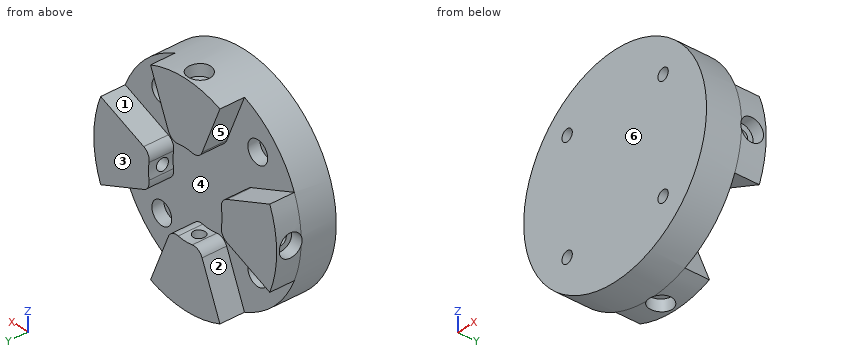
```python
from build123d import *

# Parameters (mm, degrees)
SKETCH1_R                                           = 30
BOSS_EXTRUDE1_DEPTH                                 = 10
CBORE_FOR_M3_HEX_SOCKET_HEAD_CAP_SCREW1_D           = 3.4
CBORE_FOR_M3_HEX_SOCKET_HEAD_CAP_SCREW1_CBORE_D     = 6.5
CBORE_FOR_M3_HEX_SOCKET_HEAD_CAP_SCREW1_CBORE_DEPTH = 3.4
BOSS_EXTRUDE2_DEPTH                                 = 7
CBORE_FOR_M3_HEX_SOCKET_HEAD_CAP_SCREW2_D           = 3.4
CBORE_FOR_M3_HEX_SOCKET_HEAD_CAP_SCREW2_DEPTH       = 18.91444561
CBORE_FOR_M3_HEX_SOCKET_HEAD_CAP_SCREW2_CBORE_D     = 6.5
CBORE_FOR_M3_HEX_SOCKET_HEAD_CAP_SCREW2_CBORE_DEPTH = 3.4
CIRPATTERN1_COUNT                                   = 4
FILLET1_R                                           = 3
CUT_EXTRUDE1_REACH                                  = 47.706
CIRPATTERN2_COUNT                                   = 4


with BuildPart() as part:
    # Sketch1 → Boss-Extrude1 (new body)
    with BuildSketch(Plane(origin=(0, 0, 0), x_dir=(1, 0, 0), z_dir=(0, 1, 0))):
        with Locations(Location((0, 0, 0), (0, 0, 270))):
            Circle(SKETCH1_R)
    extrude(amount=BOSS_EXTRUDE1_DEPTH)

    # CBORE for M3 Hex Socket Head Cap Screw1 (through all)
    with Locations(Plane(origin=(0, 10, 0), x_dir=(1, 0, 0), z_dir=(0, 1, 0))):
        with Locations((15.75, -15.75), (15.75, 15.75), (-15.75, 15.75), (-15.75, -15.75)):
            CounterBoreHole(CBORE_FOR_M3_HEX_SOCKET_HEAD_CAP_SCREW1_D / 2, CBORE_FOR_M3_HEX_SOCKET_HEAD_CAP_SCREW1_CBORE_D / 2, CBORE_FOR_M3_HEX_SOCKET_HEAD_CAP_SCREW1_CBORE_DEPTH)

    # Sketch5 → Boss-Extrude2 (add)
    with BuildSketch(Plane(origin=(0, 10, 0), x_dir=(1, 0, 0), z_dir=(0, 1, 0))):
        with BuildLine():
            ThreePointArc((4.592201188, -11.08655439), (0, -12), (-4.592201188, -11.08655439))
            Line((-4.592201188, -11.08655439), (-11.480502971, -27.716385975))
            ThreePointArc((-11.480502971, -27.716385975), (0, -30), (11.480502971, -27.716385975))
            Line((11.480502971, -27.716385975), (4.592201188, -11.08655439))
        make_face()
    boss_extrude2 = extrude(amount=BOSS_EXTRUDE2_DEPTH)

    # CBORE for M3 Hex Socket Head Cap Screw2
    with Locations(Plane.XY.offset(30)):
        with Locations((0, 13)):
            cbore_for_m3_hex_socket_head_cap_screw2 = CounterBoreHole(CBORE_FOR_M3_HEX_SOCKET_HEAD_CAP_SCREW2_D / 2, CBORE_FOR_M3_HEX_SOCKET_HEAD_CAP_SCREW2_CBORE_D / 2, CBORE_FOR_M3_HEX_SOCKET_HEAD_CAP_SCREW2_CBORE_DEPTH, depth=CBORE_FOR_M3_HEX_SOCKET_HEAD_CAP_SCREW2_DEPTH)

    # CirPattern1: Boss-Extrude2, CBORE for M3 Hex Socket Head Cap Screw2 ×4 about axis
    cirpattern1_axis = Axis((0, 0, 0), (0, 1, 0))
    add([boss_extrude2.rotate(cirpattern1_axis, i * 360 / CIRPATTERN1_COUNT) for i in range(1, CIRPATTERN1_COUNT)])
    add([cbore_for_m3_hex_socket_head_cap_screw2.rotate(cirpattern1_axis, i * 360 / CIRPATTERN1_COUNT) for i in range(1, CIRPATTERN1_COUNT)], mode=Mode.SUBTRACT)

    # Fillet1
    fillet1_edges = [part.edges().sort_by_distance(p)[0] for p in [
        (4.592201188, 13.5, 11.08655439),
        (-4.592201188, 13.5, 11.08655439),
        (11.08655439, 13.5, -4.592201188),
        (11.08655439, 13.5, 4.592201188),
        (-4.592201188, 13.5, -11.08655439),
        (4.592201188, 13.5, -11.08655439),
        (-11.08655439, 13.5, 4.592201188),
        (-11.08655439, 13.5, -4.592201188),
    ]]
    fillet(fillet1_edges, radius=FILLET1_R)

    # Cut-Extrude1: up to this face of the body (flat: up to its plane)
    cut_extrude1_end = Plane(part.part.faces().sort_by_distance((0, 10, 0))[0])
    # Sketch8 → Cut-Extrude1 (cut, up to the picked face)
    with BuildSketch(Plane(origin=(0, 17, 0), x_dir=(1, 0, 0), z_dir=(0, 1, 0)), mode=Mode.PRIVATE) as cut_extrude1_sk1:
        with BuildLine():
            Line((-13.616468974, -5.531886901), (-27.754500338, -11.388051237))
            ThreePointArc((-27.754500338, -11.388051237), (-27.735481678, -11.434292985), (-27.716385975, -11.480502971))
            Line((-27.716385975, -11.480502971), (-13.578200631, -5.624274854))
            ThreePointArc((-13.578200631, -5.624274854), (-12.084036828, -4.273447521), (-11.781000742, -2.282109005))
            ThreePointArc((-11.781000742, -2.282109005), (-12, 0), (-11.781000742, 2.282109005))
            ThreePointArc((-11.781000742, 2.282109005), (-12.084036828, 4.273447521), (-13.578200631, 5.624274854))
            Line((-13.578200631, 5.624274854), (-27.716385975, 11.480502971))
            ThreePointArc((-27.716385975, 11.480502971), (-27.735481678, 11.434292985), (-27.754500338, 11.388051237))
            Line((-27.754500338, 11.388051237), (-13.616468974, 5.531886901))
            ThreePointArc((-13.616468974, 5.531886901), (-12.172110631, 4.226087145), (-11.879175748, 2.30112658))
            ThreePointArc((-11.879175748, 2.30112658), (-12.1, 0), (-11.879175748, -2.30112658))
            ThreePointArc((-11.879175748, -2.30112658), (-12.172110631, -4.226087145), (-13.616468974, -5.531886901))
        make_face()
    cut_extrude1_tool1 = split(extrude(cut_extrude1_sk1.sketch, amount=-CUT_EXTRUDE1_REACH, mode=Mode.PRIVATE), bisect_by=cut_extrude1_end, keep=Keep.BOTH, mode=Mode.PRIVATE)
    cut_extrude1 = cut_extrude1_tool1.solids().sort_by(Axis((-12.147448, 17, 4.239349), (0, -1, 0)))[0]
    add(cut_extrude1, mode=Mode.SUBTRACT)

    # CirPattern2: Cut-Extrude1 ×4 about axis
    cirpattern2_axis = Axis((0, 0, 0), (0, 1, 0))
    for i in range(1, CIRPATTERN2_COUNT):
        add(cut_extrude1.rotate(cirpattern2_axis, i * 360 / CIRPATTERN2_COUNT), mode=Mode.SUBTRACT)


solid = part.part
```
For this review, take the finished solid that the model builds, in its own axes (mm). Face numbers are marked on the shaded views. A direction names the side the tool comes from. Coordinates: 2 decimals unless noted, no trailing zeros. Order: outer loops, then holes, each group sorted by start corner. A loop starts at its lowest first (then second) coordinate and runs counter-clockwise, first axis right, second up. Notation, with made-up numbers: (-2, 37.5) -> (45, 37.5) arc R28 cw to (45, 74.5) -> close; hole circle Ø3 at (-13, -23). An arc over 180 degrees is marked (long way). Answer as CSV lines item,"result".
Q1. For the marked faces 4, 5 and 6, list the 3-axis set-ups (+Z, -Z, +X, -X, +Y, -Y) from which the entire face can be reached by the end or side of a thin tool; tool diameter is ignored.
Model answer:
face 4,"+Y"
face 5,"-X, +Y"
face 6,"+Z, -Z, +X, -X, -Y"
Q2. Clearance check with flat-ended pins moving along their axes: pin 1 Ø6 at (x, y) = (13.5, 12) entering from -Z; pin 2 Ø2 at (y, z) = (14, -0.5) entering from -X; pin 3 Ø2 at (y, z) = (13, 0) entering from +X; pin 4 Ø4 at (x, y) = (0, 13) entering from -Z. State where each tip first meets the part, or that it passes through.
Model answer:
pin 1,"stops at z = -28.1"
pin 2,"stops at x = -26.6"
pin 3,"passes through"
pin 4,"stops at z = -26.6"
Q3. We need section C-C (x = 0). State the section outline as (y, z) points, plus the area to 3 significant figures.
Model answer:
outline,"(0, -30) -> (9.75, -30) -> (9.75, -26.6) -> (11.3, -26.6) -> (11.3, -12.1) -> (10, -12.1) -> (10, 12.1) -> (11.3, 12.1) -> (11.3, 26.6) -> (9.75, 26.6) -> (9.75, 30) -> (0, 30) -> close; (14.7, -26.6) -> (16.25, -26.6) -> (16.25, -30) -> (17, -30) -> (17, -12.1) -> (14.7, -12.1) -> close; (14.7, 12.1) -> (17, 12.1) -> (17, 30) -> (16.25, 30) -> (16.25, 26.6) -> (14.7, 26.6) -> close"
area,"708 mm2"
Q4. We need section B-B (y = 3.5). State the section outline as (x, z) points.
Model answer:
outline,"circle Ø60 at (0, 0); hole circle Ø3.4 at (-15.75, -15.75); hole circle Ø3.4 at (-15.75, 15.75); hole circle Ø3.4 at (15.75, -15.75); hole circle Ø3.4 at (15.75, 15.75)"
Q5. We need section D-D (x = -15.75). State the section outline as (y, z) points, plus the area to 3 significant figures.
Model answer:
outline,"(0, -25.53) -> (10, -25.53) -> (10, -19) -> (6.6, -19) -> (6.6, -17.45) -> (0, -17.45) -> close; (0, -14.05) -> (6.6, -14.05) -> (6.6, -12.5) -> (10, -12.5) -> (10, -6.42) -> (17, -6.42) -> (17, 6.42) -> (10, 6.42) -> (10, 12.5) -> (6.6, 12.5) -> (6.6, 14.05) -> (0, 14.05) -> close; (0, 17.45) -> (6.6, 17.45) -> (6.6, 19) -> (10, 19) -> (10, 25.53) -> (0, 25.53) -> close; hole circle Ø3.4 at (13, 0)"
area,"502 mm2"
Q6. Wall thickness on line 1 along Y through (x, z) = (0, 19); line 2 along Y through (x, z) = (27.8, 0); line 3 along Z through (x, y) = (-15.75, 2.5): over which ranges is each line inside the solid? List them lowest first. Write a range as [from, to].
Model answer:
line 1,"y = [0, 11.3], [14.7, 17]"
line 2,"y = [0, 9.75], [16.25, 17]"
line 3,"z = [-25.53, -17.45], [-14.05, 14.05], [17.45, 25.53]"
Q7. We need section A-A (z = 0). State the section outline as (x, y) points.
Model answer:
outline,"(-30, 0) -> (30, 0) -> (30, 9.75) -> (26.6, 9.75) -> (26.6, 11.3) -> (12.1, 11.3) -> (12.1, 10) -> (-12.1, 10) -> (-12.1, 11.3) -> (-26.6, 11.3) -> (-26.6, 9.75) -> (-30, 9.75) -> close; (-30, 16.25) -> (-26.6, 16.25) -> (-26.6, 14.7) -> (-12.1, 14.7) -> (-12.1, 17) -> (-30, 17) -> close; (12.1, 14.7) -> (26.6, 14.7) -> (26.6, 16.25) -> (30, 16.25) -> (30, 17) -> (12.1, 17) -> close"
Q8. Draft analysis for pull direction Z (two halves, no side actions). For the marked faces 1, 2 and 3, state which applies: released by +Z, released by -Z, zero draft, split by the parting line, or undercut.
Model answer:
face 1,"released by +Z"
face 2,"undercut"
face 3,"zero draft"
